Verification items for the finished model (mm, model axes). Give positions to 0.01 mm unless a question says otherwise; leave off trailing zeros. Loops run counter-clockwise (first coordinate to the right, second up) from the corner with the lowest first, then second, coordinate; pieces in that order, holes last. Notation, with made-up numbers: (-23, 29) - (4, 29) arc R19 cw to (4, 59) - close; hole circle Ø7 at (-14.5, -35). An arc over 180 degrees is marked (long way). Answer in a Markdown table with one row per item.
```python
from build123d import *

# Parameters (mm, degrees)
SKIZZE1_R                       = 1.65
AUFSATZ_LINEAR_AUSTRAGEN1_DEPTH = 5


with BuildPart() as part:
    # Skizze1 → Aufsatz-Linear austragen1 (new body)
    with BuildSketch(Plane.XY):
        with BuildLine():
            Line((-3, 0.83853083), (-16.032249001, -20.637950845))
            ThreePointArc((-16.032249001, -20.637950845), (-15.044424487, -24.79244425), (-10.903217231, -23.750323726))
            Line((-10.903217231, -23.750323726), (2.584887481, -1.522615089))
            ThreePointArc((2.584887481, -1.522615089), (2.894361971, -0.789093643), (3, 0))
            Line((3, 0), (3, 30))
            ThreePointArc((3, 30), (0, 33), (-3, 30))
            Line((-3, 30), (-3, 0.83853083))
        make_face()
        Circle(SKIZZE1_R, mode=Mode.SUBTRACT)
        with Locations((-13.488104712, -22.227708637)):
            Circle(SKIZZE1_R, mode=Mode.SUBTRACT)
    extrude(amount=AUFSATZ_LINEAR_AUSTRAGEN1_DEPTH)


solid = part.part
```
Q1. Thickness scan on line 1 (Y direction, x = -0.5, z = 1.9); line 2 (X direction, y = 27, z = 4); line 3 (Y direction, x = 0, z = 2). Record the ranges inside material, lowest first.
Completed:
| item | result |
|---|---|
| line 1 | -6.61 to -1.57, 1.57 to 32.96 |
| line 2 | -3 to 3 |
| line 3 | -5.78 to -1.65, 1.65 to 33 |
Q2. Sectioned sample at A-A (x = 0). Record the cut outline in (y, z), and give its area (3 significant figures).
Completed:
| item | result |
|---|---|
| outline | (-5.78, 0) - (-1.65, 0) - (-1.65, 5) - (-5.78, 5) - close; (1.65, 0) - (33, 0) - (33, 5) - (1.65, 5) - close |
| area | 177 mm^2 |
Q3. Sectioned sample at D-D (x = -12.75). Record the cut outline in (y, z).
Completed:
| item | result |
|---|---|
| outline | (-25.14, 0) - (-23.7, 0) - (-23.7, 5) - (-25.14, 5) - close; (-20.75, 0) - (-15.23, 0) - (-15.23, 5) - (-20.75, 5) - close |
Q4. Go/stop test with flat-tipped pins: P1, Ø3, axis at x = -6.5, z = 1, coming from the -Y side; P2, Ø2, axis at x = -13, z = 4, coming from the +Y side; P3, Ø1.5, axis at x = -5, y = 9, coming from the +Z side; P4, Ø2.5, axis at y = 16, z = 1.5, coming from the -X side. Record where each tip stops, or that it passes through.
Completed:
| item | result |
|---|---|
| P1 | y = -18.97 |
| P2 | y = -13.99 |
| P3 | through |
| P4 | x = -3 |
Q5. Sectioned sample at C-C (y = 15.5). Record the cut outline in (x, z), and give its area (3 significant figures).
Completed:
| item | result |
|---|---|
| outline | (-3, 0) - (3, 0) - (3, 5) - (-3, 5) - close |
| area | 30.0 mm^2 |
Q6. Draft check along Y on faces 1 (the face through (-13.7, -20.59, 2.46)), 2 (the face through (-15.1, -24.76, 2.46)), 3 (the face through (-3, 16, 2)). Enter one of: +Y half, -Y half, draft (parallel to the pull), parting line (faces both ways), or undercut.
Completed:
| item | result |
|---|---|
| face 1 | undercut |
| face 2 | parting line |
| face 3 | draft |
Q7. Sectioned sample at B-B (z = 2.6). Record the cut outline in (x, y).
Completed:
| item | result |
|---|---|
| outline | (-16.03, -20.64) arc R3 ccw (long way) to (-10.9, -23.75) - (2.58, -1.52) arc R3 ccw to (3, 0) - (3, 30) arc R3 ccw to (-3, 30) - (-3, 0.84) - close; hole circle Ø3.3 at (-13.49, -22.23); hole circle Ø3.3 at (0, 0) |
